Could you check a few things on this model? Use its own coordinates, in mm. A direction names the side the tool comes from. Coordinates: 2 decimals unless noted, no trailing zeros. Loops run counter-clockwise (first coordinate to the right, second up) from the corner with the lowest first, then second, coordinate; pieces in that order, holes last. Notation, with made-up numbers: M -18.5,15.5 L 35.5,15.5 A28 cw 35.5,36.5 Z; hole C 86,-22 d4. An arc over 180 degrees is marked long. Write each question's results on one line, items separated by ' | '.
```python
from build123d import *

# Parameters (mm, degrees)
CROQUIS2_W                         = 55.5
CROQUIS2_H                         = 12
BRIDA_BASE1_DEPTH                  = 1.5
BRIDA_DE_ARISTA1_STRIP_W           = 7.4732
BRIDA_DE_ARISTA1_STRIP_H           = 1.5
BRIDA_DE_ARISTA1_STRIP_CUT_DEPTH   = 12
BRIDA_DE_ARISTA1_STRIP_2_W         = 7.4732
BRIDA_DE_ARISTA1_STRIP_2_H         = 1.5
BRIDA_DE_ARISTA1_STRIP_CUT_2_DEPTH = 12
BRIDA_DE_ARISTA1_DEPTH             = 12
BRIDA_DE_ARISTA1_BEND_DEPTH        = 12
SALIENTE_EXTRUIR1_DEPTH            = 1.5
SALIENTE_EXTRUIR2_START            = -1.5
SALIENTE_EXTRUIR2_DEPTH            = 1.5
CORTAR_EXTRUIR2_REACH              = 61.835
CROQUIS17_R                        = 4
REDONDEO1_R                        = 1
REDONDEO2_R                        = 1


# Sheet-metal steps are written as plain solids
with BuildPart() as part:
    # Croquis2 → Brida base1 (new body)
    with BuildSketch(Plane(origin=(0, 0, 0), x_dir=(1, 0, 0), z_dir=(0, 1, 0))):
        Rectangle(CROQUIS2_W, CROQUIS2_H)
    extrude(amount=-BRIDA_BASE1_DEPTH)

    # Brida de arista1 strip (across the edge) → Brida de arista1 strip cut (cut)
    with BuildSketch(Plane(origin=(-27.75, -1.5, 6), x_dir=(1, 0, 0), z_dir=(0, 0, -1))):
        with Locations((-1.5, -0.75)):
            Rectangle(BRIDA_DE_ARISTA1_STRIP_W, BRIDA_DE_ARISTA1_STRIP_H)
    extrude(amount=BRIDA_DE_ARISTA1_STRIP_CUT_DEPTH, mode=Mode.SUBTRACT)

    # Brida de arista1 strip 2 (across the edge) → Brida de arista1 strip cut 2 (cut)
    with BuildSketch(Plane(origin=(27.75, -1.5, -6), x_dir=(-1, 0, 0), z_dir=(0, 0, 1))):
        with Locations((-1.5, -0.75)):
            Rectangle(BRIDA_DE_ARISTA1_STRIP_2_W, BRIDA_DE_ARISTA1_STRIP_2_H)
    extrude(amount=BRIDA_DE_ARISTA1_STRIP_CUT_2_DEPTH, mode=Mode.SUBTRACT)

    # Brida de arista1 section (across the edge) → Brida de arista1 (add)
    with BuildSketch(Plane(origin=(-27.75, -1.5, 6), x_dir=(1, 0, 0), z_dir=(0, 0, -1))):
        with BuildLine():
            Line((0, 0.7366), (0, 18.5))
            Line((0, 18.5), (1.5, 18.5))
            Line((1.5, 18.5), (1.5, 0.7366))
            ThreePointArc((1.5, 0.7366), (1.715745145, 0.215745145), (2.2366, 0))
            Line((2.2366, 0), (2.2366, -1.5))
            ThreePointArc((2.2366, -1.5), (0.655084973, -0.844915027), (0, 0.7366))
        make_face()
    extrude(amount=BRIDA_DE_ARISTA1_DEPTH)

    # Brida de arista1 section 2 (across the edge) → Brida de arista1 bend (add)
    with BuildSketch(Plane(origin=(27.75, -1.5, -6), x_dir=(-1, 0, 0), z_dir=(0, 0, 1))):
        with BuildLine():
            Line((0, 0.7366), (0, 18.5))
            Line((0, 18.5), (1.5, 18.5))
            Line((1.5, 18.5), (1.5, 0.7366))
            ThreePointArc((1.5, 0.7366), (1.715745145, 0.215745145), (2.2366, 0))
            Line((2.2366, 0), (2.2366, -1.5))
            ThreePointArc((2.2366, -1.5), (0.655084973, -0.844915027), (0, 0.7366))
        make_face()
    extrude(amount=BRIDA_DE_ARISTA1_BEND_DEPTH)

    # Croquis13 → Saliente-Extruir1 (add)
    with BuildSketch(Plane.ZY.offset(27.75)):
        with BuildLine():
            Line((-6, -20), (-10, -20))
            ThreePointArc((-10, -20), (-8.94427191, -15.527864045), (-6, -12))
            Line((-6, -12), (-6, -20))
        make_face()
        with BuildLine():
            Line((6, -20), (10, -20))
            ThreePointArc((10, -20), (8.94427191, -15.527864045), (6, -12))
            Line((6, -12), (6, -20))
        make_face()
    extrude(amount=-SALIENTE_EXTRUIR1_DEPTH)

    # Croquis16 → Saliente-Extruir2 (add)
    with BuildSketch(Plane(origin=(27.75, 0, 0), x_dir=(0, 0, -1), z_dir=(1, 0, 0)).offset(SALIENTE_EXTRUIR2_START)):
        with BuildLine():
            Line((-10, -20), (-6, -20))
            Line((-6, -20), (-6, -12))
            ThreePointArc((-6, -12), (-8.94427191, -15.527864045), (-10, -20))
        make_face()
        with BuildLine():
            Line((6, -20), (10, -20))
            ThreePointArc((10, -20), (8.94427191, -15.527864045), (6, -12))
            Line((6, -12), (6, -20))
        make_face()
    extrude(amount=SALIENTE_EXTRUIR2_DEPTH)

    # Cortar-Extruir2: up to this face of the body (flat: up to its plane)
    cortar_extruir2_end = Plane(part.part.faces().sort_by_distance((27.75, -12.121081048, 0))[0])
    # Croquis17 → Cortar-Extruir2 (cut, up to the picked face)
    with BuildSketch(Plane.ZY.offset(27.75), mode=Mode.PRIVATE) as cortar_extruir2_sk1:
        with Locations((0, -20)):
            Circle(CROQUIS17_R)
    cortar_extruir2_tool1 = split(extrude(cortar_extruir2_sk1.sketch, amount=-CORTAR_EXTRUIR2_REACH, mode=Mode.PRIVATE), bisect_by=cortar_extruir2_end, keep=Keep.BOTH, mode=Mode.PRIVATE)
    add(cortar_extruir2_tool1.solids().sort_by(Axis((-27.75, -20, 0), (1, 0, 0)))[0], mode=Mode.SUBTRACT)

    # Redondeo1
    redondeo1_edges = [part.edges().sort_by_distance(p)[0] for p in [
        (27, -20, -10),
        (27, -20, 10),
        (27, -20, 4),
        (27, -20, -4),
    ]]
    fillet(redondeo1_edges, radius=REDONDEO1_R)

    # Redondeo2
    redondeo2_edges = [part.edges().sort_by_distance(p)[0] for p in [
        (-27, -20, -4),
        (-27, -20, 4),
        (-27, -20, -10),
        (-27, -20, 10),
    ]]
    fillet(redondeo2_edges, radius=REDONDEO2_R)


solid = part.part
```
(1) Please list where these lines run through material, in increasing order: probe 1 along X at (y, z) = (-13.75, 6.5); probe 2 along Y at (x, z) = (13.5, 5.5); probe 3 along Z at (x, y) = (16.5, -1). Write a range as from..to.
Reported:
probe 1: x = -27.75..-26.25, 26.25..27.75 | probe 2: y = -1.5..0 | probe 3: z = -6..6
(2) Imagine slicing it at A-A, the plane y = -11.5. List the corners of the cut face in (x, z) for me, and give its area (3 significant figures).
Reported:
outline: M -27.75,-6 L -26.25,-6 L -26.25,6 L -27.75,6 Z; M 26.25,-6 L 27.75,-6 L 27.75,6 L 26.25,6 Z | area: 36.0 mm2
(3) Which directions (+Z, -Z, +X, -X, +Y, -Y) give clear straight access to the entire face, cutting with the end or side of a thin tool? Please do faces 1 (the flat face through (0, -1.5, 0)), 2 (the flat face through (0, -1, 6)), 3 (the cylindrical face through (27, -19.8, 4.3)).
Reported:
face 1: +Z, -Z, -Y | face 2: +Z, +X, -X, +Y | face 3: +X, -X, -Y
(4) Imagine slicing it at D-D, the plane z = -2.25. List the corners of the cut face in (x, y) for me, and give its area (3 significant figures).
Reported:
outline: M -27.75,-16.69 L -26.25,-16.69 L -26.25,-2.24 A0.74 cw -25.51,-1.5 L 25.51,-1.5 A0.74 cw 26.25,-2.24 L 26.25,-16.69 L 27.75,-16.69 L 27.75,-2.24 A2.24 ccw 25.51,0 L -25.51,0 A2.24 ccw -27.75,-2.24 Z | area: 127 mm2
(5) Imagine slicing it at C-C, the plane x = -2. List the corners of the cut face in (y, z) for me, and give its area (3 significant figures).
Reported:
outline: M -1.5,-6 L 0,-6 L 0,6 L -1.5,6 Z | area: 18.0 mm2
(6) Imagine slicing it at B-B, the plane z = 6.75. List the corners of the cut face in (x, y) for me.
Reported:
outline: M -27.75,-20 L -26.25,-20 L -26.25,-12.62 L -27.75,-12.62 Z; M 26.25,-20 L 27.75,-20 L 27.75,-12.62 L 26.25,-12.62 Z
(7) Will these pins go through, and if not, where does the flat tip stop? P1, Ø9.5, axis at x = -1.5, y = -4, coming from the +Z side; P2, Ø6, axis at x = 11.5, z = -3, coming from the +Y side; P3, Ø3, axis at x = 9.5, z = -6.5, coming from the -Y side; P4, Ø10, axis at x = 5, y = -5, coming from the -Z side.
Reported:
P1: stops at z = 6 | P2: stops at y = 0 | P3: stops at y = -1.5 | P4: stops at z = -6
(8) If we mould it in two halves opening along Z, with no side actions, what happens to faces 4 (the cylindrical face through (-27, -19.8, -4.3)), 5 (the cylindrical face through (27.01, -19.68, 9.68)), 6 (the flat face through (-26.25, -11, 0))? For each: released by +Z, released by -Z, zero draft, split by the parting line, or undercut.
Reported:
face 4: undercut | face 5: released by +Z | face 6: zero draft
